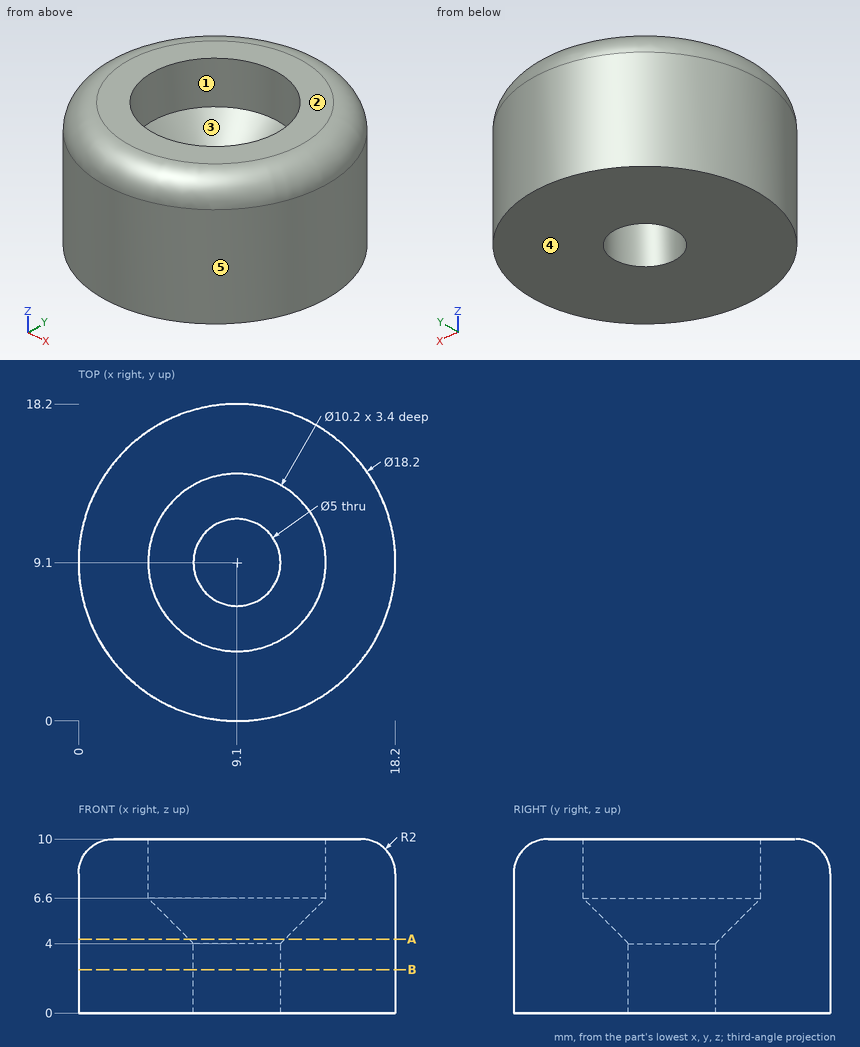
Geometry check sheet. Reference: drawing and pictorial views, mm from the part's lowest x, y, z. A direction names the side the tool comes from. Give positions to 0.01 mm unless a question says otherwise; leave off trailing zeros. Loops run counter-clockwise (first coordinate to the right, second up) from the corner with the lowest first, then second, coordinate; pieces in that order, holes last. Notation, with made-up numbers: M 58.25,-11.75 L 108.25,-11.75 A26 ccw 108.25,25.25 Z; hole C 19.5,-4 d8. An arc over 180 degrees is marked long. Use a Markdown table: item, result. Add a question column.
Q1. Scan lines: line 1 along X through (y, z) = (9.1, 2.2); line 2 along X through (y, z) = (9.1, 7.9); line 3 along Y through (x, z) = (8, 2.25) (3 decimals). Record each from-to range of solid material in increasing order. Write a range as [from, to].
Q2. Mould release check, pull along Y, two halves, no side actions. Record for the marked faces 3, 4 and 5: pulls with the +Y half, pulls with the -Y half, needs draft (parallel to the pull), parting line crosses it, or undercut.
Q3. Sectioned sample at A-A, the plane z = 4.25. Record the cut outline in (x, y), then the cut area to 3 significant figures.
Q4. Sectioned sample at B-B, the plane z = 2.5. Record the cut outline in (x, y).
Q5. Go/stop test with flat-tipped pins: pin 1 (1.5 mm diameter, centred on y = 13.5, z = 4, fed in from -X); pin 2 (9 mm diameter, centred on x = 9.1, y = 9.1, fed in from +Z); pin 3 (1 mm diameter, centred on y = 10, z = 8, fed in from +X). Record where each tip stops, or that it passes through.
Q6. Tool access check on the marked faces 1 and 2. Record the directions out of +Z, -Z, +X, -X, +Y, -Y that give a thin tool (end or side, any length) a straight path to the whole face; none if there is none.
Verdict:
| question | item | result |
|---|---|---|
| 1 | line 1 | [0, 6.6], [11.6, 18.2] |
| 1 | line 2 | [0, 4], [14.2, 18.2] |
| 1 | line 3 | [0.067, 6.855], [11.345, 18.133] |
| 2 | face 3 | undercut |
| 2 | face 4 | needs draft |
| 2 | face 5 | parting line crosses it |
| 3 | outline | C 9.1,9.1 d18.2; hole C 9.1,9.1 d5.5 |
| 3 | area | 236 mm^2 |
| 4 | outline | C 9.1,9.1 d18.2; hole C 9.1,9.1 d5 |
| 5 | pin 1 | x = 0.76 |
| 5 | pin 2 | z = 6 |
| 5 | pin 3 | x = 18.19 |
| 6 | face 1 | +Z |
| 6 | face 2 | +Z, +X, -X, +Y, -Y |
